```python
from build123d import *

# Parameters (mm, degrees)
SKETCH1_W           = 100
SKETCH1_H           = 100
BOSS_EXTRUDE1_DEPTH = 100
SKETCH2_R           = 10
CUT_EXTRUDE1_DEPTH  = 58
CHAMFER1_SIZE       = 10


with BuildPart() as part:
    # Sketch1 → Boss-Extrude1 (new body)
    with BuildSketch(Plane.XY):
        Rectangle(SKETCH1_W, SKETCH1_H)
    extrude(amount=BOSS_EXTRUDE1_DEPTH)

    # Sketch2 → Cut-Extrude1 (cut)
    with BuildSketch(Plane.XY.offset(100)):
        Circle(SKETCH2_R)
    extrude(amount=-CUT_EXTRUDE1_DEPTH, mode=Mode.SUBTRACT)

    # Chamfer1
    chamfer1_edges = [part.edges().sort_by_distance(p)[0] for p in [
        (-50, -50, 50),
    ]]
    chamfer(chamfer1_edges, length=CHAMFER1_SIZE)


solid = part.part
```
Could you check a few things on this model? Use its own coordinates, in mm. A direction names the side the tool comes from. Round coordinates to 2 decimals unless told otherwise and drop trailing zeros. Write each loop counter-clockwise with the first axis right and the second up, starting at its lowest first coordinate (ties: lowest second). Pieces come first, ordered by that corner, then holes.
(1) Suppose I cut it at A-A on z = 49. Write out the boundary of the cut face in (x, y).
Findings below:
outline: (-50, -40) - (-40, -50) - (50, -50) - (50, 50) - (-50, 50) - close; hole circle Ø20 at (0, 0)
(2) If I drill on probe 1 along Y at (x, z) = (0, 85); probe 2 along Z at (x, y) = (-6, -2); probe 3 along X at (y, z) = (-7.5, 71), over which ranges is the centre line in solid material (lowest first)?
Findings below:
probe 1: y = -50 to -10, 10 to 50
probe 2: z = 0 to 42
probe 3: x = -50 to -6.61, 6.61 to 50
(3) Which directions (+Z, -Z, +X, -X, +Y, -Y) give clear straight access to the entire face, cutting with the end or side of a thin tool? Please do faces 5 (the face through (0, 0, 42)), 6 (the face through (-1, 12, 100)).
Findings below:
face 5: +Z
face 6: +Z, +X, -X, +Y, -Y
(4) For pin 1 (22 mm diameter, centred on x = -4.5, y = 0.5, fed in from +Z), with a flat end and sliding along its axis, tell me the tip position at first contact or that it passes through.
Findings below:
pin 1: stops at z = 100
(5) Suppose I cut it at B-B on y = 0. Write out the boundary of the cut face in (x, z), and give its area (3 significant figures).
Findings below:
outline: (-50, 0) - (50, 0) - (50, 100) - (10, 100) - (10, 42) - (-10, 42) - (-10, 100) - (-50, 100) - close
area: 8,840 mm2
(6) Thinking about a two-plate mould opening in Y: for faces 1 (the face through (4, -50, 49)), 2 (the face through (-1, 50, 49)), 3 (the face through (-2.17, -9.76, 71.41)), 4 (the face through (-50, 4, 49)), which applies, +Y half, -Y half, draft (parallel to the pull), parting line (faces both ways), or undercut?
Findings below:
face 1: -Y half
face 2: +Y half
face 3: undercut
face 4: draft
